Geometry check sheet. Reference: the model listing, model coordinates, mm. A direction names the side the tool comes from. Give positions to 0.01 mm unless a question says otherwise; leave off trailing zeros. Order: outer loops, then holes, each group sorted by start corner. A loop starts at its lowest first (then second) coordinate and runs counter-clockwise, first axis right, second up. Notation, with made-up numbers: M -29.5,-40 L -5.5,-40 A30 ccw -5.5,-17 Z; hole C 72,15 d10. An arc over 180 degrees is marked long. Put each result on its own line as item: value. Start each with the question number.
Q1. Section check A-A on z = 1.5. Record the cut outline in (x, y), then the cut area to 3 significant figures.
Q2. Go/stop test with flat-tipped pins: pin 1 (0.9 mm diameter, centred on x = -45.5, z = 3, fed in from -Y); pin 2 (3 mm diameter, centred on x = -30.5, z = 7, fed in from -Y); pin 3 (2 mm diameter, centred on x = -43.5, z = 5, fed in from -Y). Record where each tip stops, or that it passes through.
Q3. Section check B-B on x = 1.5. Record the cut outline in (y, z).
Q4. Section check C-C on y = 55. Record the cut outline in (x, z), then the cut area to 3 significant figures.
Q5. Material ranges on L1, parallel to X at y = 68.75, z = 4.5; L2, parallel to Y at x = 43, z = 5; L3, parallel to X at y = 46.25, z = 2, recorded low to high.
Q6. Access from +Z, -Z, +X, -X, +Y, -Y to the whole of each face (thin tool, end or side, straight path). Record for faces 1 (the flat face through (46, 65.63, 4)), 2 (the flat face through (-46, 65.63, 4)), 3 (the flat face through (47.75, 69, 4)), 4 (the flat face through (44.75, 68, 4)).
```python
from build123d import *

# Parameters (mm, degrees)
BOSS_EXTRU_1_DEPTH = 8


with BuildPart() as part:
    # Esquisse2 → Boss.-Extru.1 (new body)
    with BuildSketch(Plane.XY):
        with BuildLine():
            Line((-47.75, 65.629607354), (-44.75, 65.629607354))
            Line((-44.75, 65.629607354), (-44.75, 69.468928374))
            Line((-44.75, 69.468928374), (-40.831689929, 69.468928374))
            Line((-40.831689929, 69.468928374), (-5.991442082, 45.011388011))
            ThreePointArc((-5.991442082, 45.011388011), (0, 48), (5.991442082, 45.011388011))
            Line((5.991442082, 45.011388011), (40.831689929, 69.468928374))
            Line((40.831689929, 69.468928374), (44.75, 69.468928374))
            Line((44.75, 69.468928374), (44.75, 65.629607354))
            Line((44.75, 65.629607354), (47.75, 65.629607354))
            Line((47.75, 65.629607354), (47.75, 72.468928374))
            Line((47.75, 72.468928374), (-47.75, 72.468928374))
            Line((-47.75, 72.468928374), (-47.75, 65.629607354))
        make_face()
    extrude(amount=BOSS_EXTRU_1_DEPTH)


solid = part.part
```
Results found:
1. outline: M -47.75,65.63 L -44.75,65.63 L -44.75,69.47 L -40.83,69.47 L -5.99,45.01 A7.5 cw 5.99,45.01 L 40.83,69.47 L 44.75,69.47 L 44.75,65.63 L 47.75,65.63 L 47.75,72.47 L -47.75,72.47 Z
1. area: 1,430 mm^2
2. pin 1: stops at y = 65.63
2. pin 2: stops at y = 61.16
2. pin 3: stops at y = 69.47
3. outline: M 47.85,0 L 72.47,0 L 72.47,8 L 47.85,8 Z
4. outline: M -20.22,0 L 20.22,0 L 20.22,8 L -20.22,8 Z
4. area: 324 mm^2
5. L1: x = -47.75 to -44.75, -39.81 to 39.81, 44.75 to 47.75
5. L2: y = 69.47 to 72.47
5. L3: x = -7.76 to -4.82, 4.82 to 7.76
6. face 1: +Z, -Z, +X, -Y
6. face 2: +Z, -Z, -X, -Y
6. face 3: +Z, -Z, +X, +Y, -Y
6. face 4: +Z, -Z, -Y
